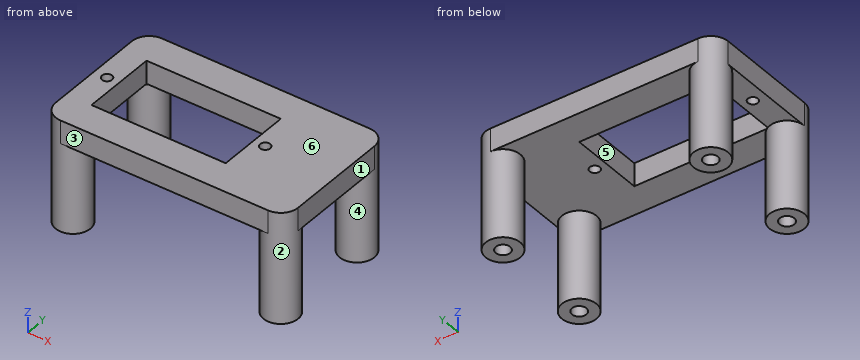
Solid Edge part; units mm, degrees
sketch "Sketch1" plane through (0, 0, 0) normal (0, 0, 1) x (1, 0, 0)
  line L0 (-18, 12) -> (18, 12)
  line L1 (21, 9) -> (21, -9)
  line L2 (-18, -12) -> (18, -12)
  line L3 (-21, 9) -> (-21, -9)
  arc A0 (18, 12) -> (21, 9) centre (18, 9) cw
  arc A1 (21, -9) -> (18, -12) centre (18, -9) cw
  arc A2 (-18, -12) -> (-21, -9) centre (-18, -9) cw
  arc A3 (-21, 9) -> (-18, 12) centre (-18, 9) cw
  circle A4 centre (8.7, 0) radius 0.875
  circle A5 centre (-18.7, 0) radius 0.875
  line L4 (6.625, -6.5) -> (-16.625, -6.5)
  line L5 (-16.625, -6.5) -> (-16.625, 6.5)
  line L6 (-16.625, 6.5) -> (6.625, 6.5)
  line L7 (6.625, 6.5) -> (6.625, -6.5)
extrude "Protrusion1" add sketch "Sketch1" along normal blind 4
sketch "Sketch2" plane through (0, 0, 0) normal (0, 0, -1) x (1, 0, 0)
  circle A0 centre (-18, 9) radius 3
  circle A1 centre (18, 9) radius 3
  circle A2 centre (-18, -9) radius 3
  circle A3 centre (18, -9) radius 3
extrude "ExtrudedProtrusion_3" add sketch "Sketch2" along normal blind 15.25
sketch "Sketch3" plane through (18, -9, -15.25) normal (0, 0, -1) x (1, 0, 0)
  circle A0 centre (0, 0) radius 1.25
  circle A1 centre (0, -18) radius 1.25
  circle A2 centre (-36, -18) radius 1.25
  circle A3 centre (-36, 0) radius 1.25
extrude "ExtrudedCutout_1" cut sketch "Sketch3" against normal blind 10
Design review of the part built by this model. Coordinates are the model's own, in mm. Face numbers are marked on the shaded views. A direction names the side the tool comes from. Coordinates: 2 decimals unless noted, no trailing zeros. Loops run counter-clockwise (first coordinate to the right, second up) from the corner with the lowest first, then second, coordinate; pieces in that order, holes last.
Item 1: Draft analysis for pull direction X (two halves, no side actions). For the marked faces 1, 2 and 3, state which applies: pulls with the +X half, pulls with the -X half, needs draft (parallel to the pull), parting line crosses it, or undercut.
Completed:
face 1: pulls with the +X half
face 2: undercut
face 3: needs draft
Item 2: Wall thickness on L1, parallel to Y at x = 18, z = -7.75; L2, parallel to X at y = -9, z = -8; L3, parallel to Y at x = -16.5, z = 0.5: over which ranges is each line inside the solid? List them lowest first.
Completed:
L1: y = -12 to -10.25, -7.75 to -6, 6 to 7.75, 10.25 to 12
L2: x = -21 to -19.25, -16.75 to -15, 15 to 16.75, 19.25 to 21
L3: y = -12 to -6.5, 6.5 to 12
Item 3: For the marked faces 4, 5 and 6, list the 3-axis set-ups (+Z, -Z, +X, -X, +Y, -Y) from which the entire face can be reached by the end or side of a thin tool; tool diameter is ignored.
Completed:
face 4: -Z
face 5: +Z, -Z
face 6: +Z, +X, -X, +Y, -Y
Item 4: Add section B-B (y = 0). Write out the cut boundary in (x, z) (3 decimals).
Completed:
outline: (-21, 0) - (-19.575, 0) - (-19.575, 4) - (-21, 4) - close; (-17.825, 0) - (-16.625, 0) - (-16.625, 4) - (-17.825, 4) - close; (6.625, 0) - (7.825, 0) - (7.825, 4) - (6.625, 4) - close; (9.575, 0) - (21, 0) - (21, 4) - (9.575, 4) - close
Item 5: Add section D-D (y = -5). Write out the cut boundary in (x, z) (3 decimals).
Completed:
outline: (-21, 0) - (-16.625, 0) - (-16.625, 4) - (-21, 4) - close; (6.625, 0) - (21, 0) - (21, 4) - (6.625, 4) - close
Item 6: Clearance check with flat-ended pins moving along their axes: pin 1 (0.8 mm diameter, centred on x = -18, y = -8.5, fed in from -Z); pin 2 (1.6 mm diameter, centred on x = 8.7, y = 0, fed in from +Z); pin 3 (2 mm diameter, centred on x = -18, y = -1, fed in from -Z). State where each tip first meets the part, or that it passes through.
Completed:
pin 1: stops at z = -5.25
pin 2: passes through
pin 3: stops at z = 0
Item 7: Add section A-A (z = -9). Write out the cut boundary in (x, y), and give its area (3 significant figures).
Completed:
outline: circle Ø6 at (-18, -9); circle Ø6 at (-18, 9); circle Ø6 at (18, -9); circle Ø6 at (18, 9); hole circle Ø2.5 at (-18, -9); hole circle Ø2.5 at (-18, 9); hole circle Ø2.5 at (18, -9); hole circle Ø2.5 at (18, 9)
area: 93.5 mm2
Item 8: Add section C-C (x = -10). Write out the cut boundary in (y, z).
Completed:
outline: (-12, 0) - (-6.5, 0) - (-6.5, 4) - (-12, 4) - close; (6.5, 0) - (12, 0) - (12, 4) - (6.5, 4) - close
